from build123d import *

# Parameters (mm, degrees)
SKETCH1_W           = 8.5
SKETCH1_H           = 8.5
BOSS_EXTRUDE1_DEPTH = 5
SKETCH2_W           = 8.5
SKETCH2_H           = 8.5
BOSS_EXTRUDE2_DEPTH = 2
SKETCH3_R           = 1.5
CUT_EXTRUDE1_DEPTH  = 2
SKETCH4_W           = 52
SKETCH4_H           = 8.5
BOSS_EXTRUDE3_DEPTH = 3
SKETCH5_W           = 7
SKETCH5_H           = 8.5
BOSS_EXTRUDE4_DEPTH = 8.5
CUT_EXTRUDE2_DEPTH  = 5
SKETCH7_R           = 1.5
CUT_EXTRUDE3_DEPTH  = 5
SKETCH8_R           = 1.5
BOSS_EXTRUDE5_DEPTH = 2.5
SKETCH9_R           = 1.5
BOSS_EXTRUDE6_DEPTH = 2.5
SKETCH10_W          = 8.5
SKETCH10_H          = 8.5
BOSS_EXTRUDE7_DEPTH = 1
SKETCH11_W          = 8.5
SKETCH11_H          = 8.5
BOSS_EXTRUDE8_DEPTH = 1
CUT_EXTRUDE4_DEPTH  = 0.5
CUT_EXTRUDE5_DEPTH  = 0.5


with BuildPart() as part:
    # Sketch1 → Boss-Extrude1 (new body)
    with BuildSketch(Plane(origin=(0, 0, 0), x_dir=(0, 0, -1), z_dir=(1, 0, 0))):
        Rectangle(SKETCH1_W, SKETCH1_H)
        Polygon((1.705, 2.953146627), (-1.705, 2.953146627), (-3.41, 0), (-1.705, -2.953146627), (1.705, -2.953146627), (3.41, 0), align=None, mode=Mode.SUBTRACT)
    extrude(amount=BOSS_EXTRUDE1_DEPTH)

    # Sketch2 → Boss-Extrude2 (add)
    with BuildSketch(Plane.ZY):
        Rectangle(SKETCH2_W, SKETCH2_H)
    extrude(amount=BOSS_EXTRUDE2_DEPTH)

    # Sketch3 → Cut-Extrude1 (cut)
    with BuildSketch(Plane(origin=(0, 0, 0), x_dir=(0, 0, -1), z_dir=(1, 0, 0))):
        Circle(SKETCH3_R)
    extrude(amount=-CUT_EXTRUDE1_DEPTH, mode=Mode.SUBTRACT)

    # Sketch4 → Boss-Extrude3 (add)
    with BuildSketch(Plane.XZ.offset(4.25)):
        with Locations((24, 0)):
            Rectangle(SKETCH4_W, SKETCH4_H)
    extrude(amount=BOSS_EXTRUDE3_DEPTH)

    # Sketch5 → Boss-Extrude4 (add)
    with BuildSketch(Plane(origin=(0, -4.25, 0), x_dir=(1, 0, 0), z_dir=(0, 1, 0))):
        with Locations((46.5, 0)):
            Rectangle(SKETCH5_W, SKETCH5_H)
    extrude(amount=BOSS_EXTRUDE4_DEPTH)

    # Sketch6 → Cut-Extrude2 (cut)
    with BuildSketch(Plane.ZY.offset(-43)):
        Polygon((3.41, 0), (1.705, 2.953146627), (-1.705, 2.953146627), (-3.41, 0), (-1.705, -2.953146627), (1.705, -2.953146627), align=None)
    extrude(amount=-CUT_EXTRUDE2_DEPTH, mode=Mode.SUBTRACT)

    # Sketch7 → Cut-Extrude3 (cut)
    with BuildSketch(Plane.ZY.offset(-48)):
        Circle(SKETCH7_R)
    extrude(amount=-CUT_EXTRUDE3_DEPTH, mode=Mode.SUBTRACT)

    # Sketch8 → Boss-Extrude5 (add)
    with BuildSketch(Plane(origin=(0, 0, 0), x_dir=(0, 0, -1), z_dir=(1, 0, 0))):
        Polygon((-1.705, 2.953146627), (-3.41, 0), (-1.705, -2.953146627), (1.705, -2.953146627), (3.41, 0), (1.705, 2.953146627), align=None)
        Circle(SKETCH8_R, mode=Mode.SUBTRACT)
    extrude(amount=BOSS_EXTRUDE5_DEPTH)

    # Sketch9 → Boss-Extrude6 (add)
    with BuildSketch(Plane.ZY.offset(-48)):
        Polygon((3.41, 0), (1.705, 2.953146627), (-1.705, 2.953146627), (-3.41, 0), (-1.705, -2.953146627), (1.705, -2.953146627), align=None)
        Circle(SKETCH9_R, mode=Mode.SUBTRACT)
    extrude(amount=BOSS_EXTRUDE6_DEPTH)

    # Sketch10 → Boss-Extrude7 (add)
    with BuildSketch(Plane(origin=(5, 0, 0), x_dir=(0, 0, -1), z_dir=(1, 0, 0))):
        Rectangle(SKETCH10_W, SKETCH10_H)
        Polygon((3.41, 0), (1.705, 2.953146627), (-1.705, 2.953146627), (-3.41, 0), (-1.705, -2.953146627), (1.705, -2.953146627), align=None, mode=Mode.SUBTRACT)
    extrude(amount=BOSS_EXTRUDE7_DEPTH)

    # Sketch11 → Boss-Extrude8 (add)
    with BuildSketch(Plane.ZY.offset(-43)):
        Rectangle(SKETCH11_W, SKETCH11_H)
        Polygon((-3.41, 0), (-1.705, -2.953146627), (1.705, -2.953146627), (3.41, 0), (1.705, 2.953146627), (-1.705, 2.953146627), align=None, mode=Mode.SUBTRACT)
    extrude(amount=BOSS_EXTRUDE8_DEPTH)

    # Sketch12 → Cut-Extrude4 (cut)
    with BuildSketch(Plane(origin=(2.5, 0, 0), x_dir=(0, 0, -1), z_dir=(1, 0, 0))):
        Polygon((1.705, -2.953146627), (3.41, 0), (1.705, 2.953146627), (-1.705, 2.953146627), (-3.41, 0), (-1.705, -2.953146627), align=None)
    extrude(amount=-CUT_EXTRUDE4_DEPTH, mode=Mode.SUBTRACT)

    # Sketch13 → Cut-Extrude5 (cut)
    with BuildSketch(Plane.ZY.offset(-45.5)):
        Polygon((1.705, 2.953146627), (-1.705, 2.953146627), (-3.41, 0), (-1.705, -2.953146627), (1.705, -2.953146627), (3.41, 0), align=None)
    extrude(amount=-CUT_EXTRUDE5_DEPTH, mode=Mode.SUBTRACT)


solid = part.part
Geometry check sheet. Reference: the model listing, model coordinates, mm. A direction names the side the tool comes from. Round coordinates to 2 decimals unless told otherwise and drop trailing zeros. Order: outer loops, then holes, each group sorted by start corner. A loop starts at its lowest first (then second) coordinate and runs counter-clockwise, first axis right, second up. Notation, with made-up numbers: (9, 25) - (67, 25) arc R35 ccw to (67, 62) - close; hole circle Ø9 at (7, 89.25). An arc over 180 degrees is marked (long way). One line per question, with ' | ' between items. Start each with the question number.
(1) Sectioned sample at B-B on y = -0.5. Record the cut outline in (x, z).
(2) Release check for a two-part mould opening along X. For faces 4 (the flat face through (44, 2.953, 0)), 5 (the flat face through (-2, -1.4, -1)), 6 (the flat face through (24, -5, -4.25)) record: released by +X, released by -X, zero draft, split by the parting line, or undercut.
(3) Sectioned sample at C-C on x = 16.5. Record the cut outline in (y, z).
(4) Sectioned sample at A-A on z = 0. Record the cut outline in (x, y), and give its area (3 significant figures).
(5) Access from +Z, -Z, +X, -X, +Y, -Y to the whole of each face (thin tool, end or side, straight path). Record for faces 1 (the flat face through (44.028, -1.497, 2.546)), 2 (the flat face through (24, -7.25, 0)), 3 (the flat face through (24, -4.25, 0)).
(6) Depth check by flat-ended pin: pin 1 Ø3 at (x, z) = (20.5, -3) entering from +Y; pin 2 Ø2.5 at (y, z) = (0, 0) entering from +X. Enter the tip coordinate at first touch or a pass-through.
(7) Thickness scan on L1, parallel to Y at x = -0.1, z = 0; L2, parallel to Z at x = 0.1, y = 0; L3, parallel to X at y = 1, z = 3.5. Record the ranges inside material, lowest first. Write a range as [from, to].
Conclusion:
1) outline: (-2, -4.25) - (6, -4.25) - (6, -3.12) - (2, -3.12) - (2, -1.41) - (-2, -1.41) - close; (-2, 1.41) - (2, 1.41) - (2, 3.12) - (6, 3.12) - (6, 4.25) - (-2, 4.25) - close; (42, -4.25) - (50, -4.25) - (50, -1.41) - (46, -1.41) - (46, -3.12) - (42, -3.12) - close; (42, 3.12) - (46, 3.12) - (46, 1.41) - (50, 1.41) - (50, 4.25) - (42, 4.25) - close
2) face 4: undercut | face 5: released by -X | face 6: zero draft
3) outline: (-7.25, -4.25) - (-4.25, -4.25) - (-4.25, 4.25) - (-7.25, 4.25) - close
4) outline: (-2, -7.25) - (50, -7.25) - (50, -1.5) - (46, -1.5) - (46, -2.95) - (42, -2.95) - (42, -4.25) - (6, -4.25) - (6, -2.95) - (2, -2.95) - (2, -1.5) - (-2, -1.5) - close; (-2, 1.5) - (2, 1.5) - (2, 2.95) - (6, 2.95) - (6, 4.25) - (-2, 4.25) - close; (42, 2.95) - (46, 2.95) - (46, 1.5) - (50, 1.5) - (50, 4.25) - (42, 4.25) - close | area: 221 mm2
5) face 1: none | face 2: +Z, -Z, +X, -X, -Y | face 3: +Z, -Z, +Y
6) pin 1: stops at y = -4.25 | pin 2: passes through
7) L1: y = [-7.25, -1.5], [1.5, 4.25] | L2: z = [-4.25, -1.5], [1.5, 4.25] | L3: x = [-2, 6], [42, 50]
